```python
from build123d import *

# Parameters (mm, degrees)
BOSS_EXTRU_1_DEPTH = 305


with BuildPart() as part:
    # Esquisse1 → Boss.-Extru.1 (new body)
    with BuildSketch(Plane.XY):
        with BuildLine():
            Line((-25.931265673, -2.76101993), (-15.181265673, -2.76101993))
            Line((-15.181265673, -2.76101993), (-15.181265673, 3.93898007))
            Line((-15.181265673, 3.93898007), (-13.453102315, 3.93898007))
            Line((-13.453102315, 3.93898007), (-9.931265673, 10.03898007))
            ThreePointArc((-9.931265673, 10.03898007), (-6.010431334, 25.012290482), (-2.089596996, 10.03898007))
            Line((-2.089596996, 10.03898007), (1.432239646, 3.93898007))
            Line((1.432239646, 3.93898007), (3.160403004, 3.93898007))
            Line((3.160403004, 3.93898007), (3.160403004, -2.76101993))
            Line((3.160403004, -2.76101993), (14.068734327, -2.76101993))
            Line((14.068734327, -2.76101993), (14.068734327, -7.76101993))
            Line((14.068734327, -7.76101993), (-25.931265673, -7.76101993))
            Line((-25.931265673, -7.76101993), (-25.931265673, -2.76101993))
        make_face()
    extrude(amount=BOSS_EXTRU_1_DEPTH)


solid = part.part
```
The listing builds one solid part. Answer for the finished solid, in the listing's coordinates (mm). A direction names the side the tool comes from. Give positions to 0.01 mm unless a question says otherwise; leave off trailing zeros. Order: outer loops, then holes, each group sorted by start corner. A loop starts at its lowest first (then second) coordinate and runs counter-clockwise, first axis right, second up. Notation, with made-up numbers: (-34, 7) -> (-23, 7) arc R22 cw to (-23, 37) -> close; hole circle Ø8 at (3.25, -25.75). An arc over 180 degrees is marked (long way). Answer as CSV lines item,"result". Start each with the question number.
Q1. Which of the six approach directions +Z, -Z, +X, -X, +Y, -Y give full straight-line access (tool end or side, diameter ignored) to faces 1 (the flat face through (14.069, -5, 150)), 2 (the flat face through (9, -2.761, 150)), 3 (the flat face through (-15.181, 1, 150))?
Q2. Determine the mould class of faces 4 (the flat face through (3.16, 1, 150)), 5 (the flat face through (-0.353, 7.032, 150.365)), 6 (the flat face through (-11.717, 6.946, 150.365)), 7 (the flat face through (-21, -2.761, 150)) for opening direction Y: pulls with the +Y half, pulls with the -Y half, needs draft (parallel to the pull), parting line crosses it, or undercut.
Q3. A cutting plane is placed at A-A (z = 83.5). Determine the outline of the cut face in (x, y).
Q4. A cutting plane is placed at B-B (x = 7). Determine the outline of the cut face in (y, z), then the cut area to 4 significant figures.
Q5. A cutting plane is placed at C-C (y = 1). Determine the outline of the cut face in (x, z), then the cut area to 3 significant figures.
Q6. Find the intervals of material crossed by L1, parallel to Y at x = -20.5, z = 238; L2, parallel to X at y = 16.5, z = 89; L3, parallel to Y at x = -2, z = 252, in increasing order.
Q7. Given pin 1 (7.5 mm diameter, centred on y = 0.5, z = 100.5, fed in from +X); pin 2 (0.5 mm diameter, centred on x = -14.5, z = 101.5, fed in from +Y); pin 3 (1.5 mm diameter, centred on x = -9, z = 34.5, fed in from +Y); pin 4 (8 mm diameter, centred on y = 7.5, z = 122.5, fed in from +X), each flat-ended and moving along its own axis, determine where each tip first touches the part or whether it passes through.
Results found:
1,face 1,"+Z, -Z, +X, +Y, -Y"
1,face 2,"+Z, -Z, +X, +Y"
1,face 3,"+Z, -Z, -X, +Y"
2,face 4,"needs draft"
2,face 5,"undercut"
2,face 6,"undercut"
2,face 7,"pulls with the +Y half"
3,outline,"(-25.93, -7.76) -> (14.07, -7.76) -> (14.07, -2.76) -> (3.16, -2.76) -> (3.16, 3.94) -> (1.43, 3.94) -> (-2.09, 10.04) arc R8 ccw (long way) to (-9.93, 10.04) -> (-13.45, 3.94) -> (-15.18, 3.94) -> (-15.18, -2.76) -> (-25.93, -2.76) -> close"
4,outline,"(-7.76, 0) -> (-2.76, 0) -> (-2.76, 305) -> (-7.76, 305) -> close"
4,area,"1,525 mm2"
5,outline,"(-15.18, 0) -> (3.16, 0) -> (3.16, 305) -> (-15.18, 305) -> close"
5,area,"5,590 mm2"
6,L1,"-7.76 to -2.76"
6,L2,"-13.99 to 1.97"
6,L3,"-7.76 to 9.88, 10.09 to 23.93"
7,pin 1,"x = 14.07"
7,pin 2,"y = 3.94"
7,pin 3,"y = 24.69"
7,pin 4,"x = 3.16"
